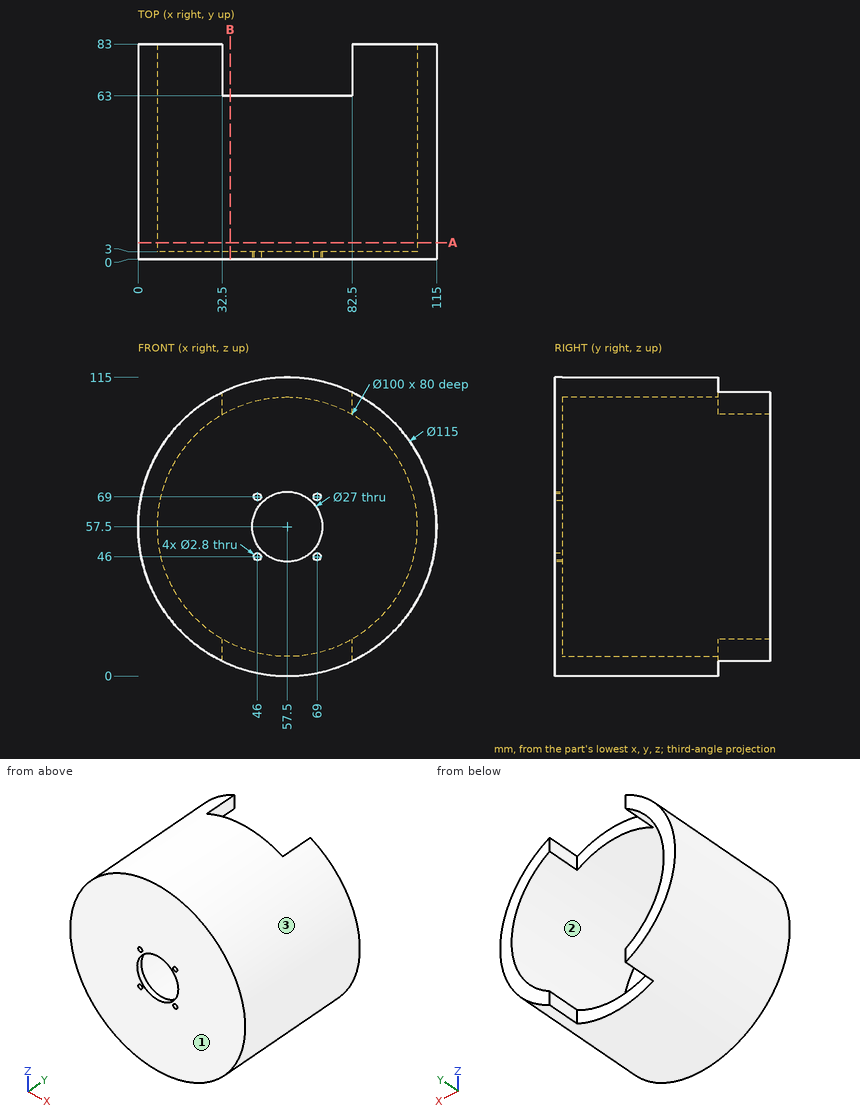
Here's the drawing with two shaded views (mm, measured from the low corner). I have some questions. Give positions to 0.01 mm unless a question says otherwise; leave off trailing zeros. Write each loop counter-clockwise with the first axis right and the second up, starting at its lowest first coordinate (ties: lowest second). Pieces come first, ordered by that corner, then holes. Notation, with made-up numbers: (0, -11.5) -> (7, -11.5) arc R15 ccw to (7, 7.5) -> close; hole circle Ø4 at (15.25, -8). An arc over 180 degrees is marked (long way). One line per item, written item: value.
Q1. Imagine slicing it at A-A on y = 6.5. Please give me the cut outline in (x, z).
Results found:
outline: circle Ø115 at (57.5, 57.5); hole circle Ø100 at (57.5, 57.5)
Q2. We'd pull the mould along Z, two halves only. Please class the marked faces 1, 2 and 3: +Z half, -Z half, draft (parallel to the pull), parting line (faces both ways), or undercut.
Results found:
face 1: draft
face 2: undercut
face 3: parting line
Q3. For P1, Ø6, axis at x = 29.5, y = 53, coming from the -Z side; P2, Ø12, axis at y = 67, z = 79.5, coming from the -X side; P3, Ø21.5, axis at x = 57.5, z = 57.5, coming from the +Y side; P4, Ø15.5, axis at x = 50, z = 110.5, coming from the +Y side, each with a flat end and sliding along its axis, tell me the tip position at first contact or that it passes through.
Results found:
P1: stops at z = 5.72
P2: stops at x = 2.27
P3: passes through
P4: stops at y = 63
Q4. Imagine slicing it at B-B on x = 35.5. Please give me the cut outline in (y, z).
Results found:
outline: (0, 4.38) -> (63, 4.38) -> (63, 12.6) -> (3, 12.6) -> (3, 102.4) -> (63, 102.4) -> (63, 110.62) -> (0, 110.62) -> close
Q5. Please list where these lines run through material, in increasing order: line 1 (X direction, y = 1, z = 46); line 2 (Y direction, x = 29, z = 32.5); line 3 (Z direction, x = 28.5, y = 18). Write a range as [from, to].
Results found:
line 1: x = [1.16, 44.6], [47.4, 50.43], [64.57, 67.6], [70.4, 113.84]
line 2: y = [0, 3]
line 3: z = [7.85, 16.77], [98.23, 107.15]
